from build123d import *

# Parameters (mm, degrees)
F0_R          = 8.875
F3_DEPTH      = 3
F3_DEPTH_BACK = 3
F4_SIZE       = 1
F5_R          = 0.5
F6_DEPTH      = 0.43


with BuildPart() as f2:
    # F0 (on Front) → F2 (revolve)
    with BuildSketch(Plane.XZ):
        with BuildLine():
            ThreePointArc((0, 10.375), (1.4661242569, 10.2708862647), (2.9028232275, 9.9606346339))
            ThreePointArc((2.9028232275, 9.9606346339), (9.4069705736, 10.9259285589), (15, 14.3833476682))
            Line((15, 14.3833476682), (3.7, 34.9606346339))
            Line((3.7, 34.9606346339), (0, 34.9606346339))
            Line((0, 34.9606346339), (0, 10.375))
        make_face()
    revolve(axis=Axis((0, 0, 0), (0, 0, 1)))

    # F0 (on Front) → F3 (join, two sides)
    with BuildSketch(Plane.XZ) as f3_sk:
        with BuildLine():
            ThreePointArc((0, 10.375), (-7.3362328548, -7.3362328548), (10.375, 0))
            ThreePointArc((10.375, 0), (8.2993197307, 6.2259069225), (2.9028232275, 9.9606346339))
            Line((2.9028232275, 9.9606346339), (0, 9.9606346339))
            Line((0, 9.9606346339), (0, 10.375))
        make_face()
        Circle(F0_R, mode=Mode.SUBTRACT)
        with BuildLine():
            Line((0, 9.9606346339), (2.9028232275, 9.9606346339))
            ThreePointArc((2.9028232275, 9.9606346339), (1.4661242569, 10.2708862647), (0, 10.375))
            Line((0, 10.375), (0, 9.9606346339))
        make_face()
    extrude(amount=F3_DEPTH)
    extrude(f3_sk.sketch, amount=-F3_DEPTH_BACK)

    # F4
    f4_edges = [f2.edges().sort_by_distance(p)[0] for p in [
        (-8.875, -3, 0),
        (-8.875, 3, 0),
    ]]
    chamfer(f4_edges, length=F4_SIZE)

    # F5 (on face) → F6 (cut)
    with BuildSketch(Plane.XY.offset(34.9606346339)):
        with BuildLine():
            ThreePointArc((0.0041443855, 1.7524251654), (-0.4908303614, 1.5473999123), (-0.6958556145, 1.0524251654))
            Line((-0.6958556145, 1.0524251654), (-0.6958556145, -1.0399995122))
            ThreePointArc((-0.6958556145, -1.0399995122), (-0.4908303614, -1.534974259), (0.0041443855, -1.7399995122))
            ThreePointArc((0.0041443855, -1.7399995122), (0.4991191323, -1.534974259), (0.7041443855, -1.0399995122))
            Line((0.7041443855, -1.0399995122), (0.7041443855, 1.0524251654))
            ThreePointArc((0.7041443855, 1.0524251654), (0.4991191323, 1.5473999123), (0.0041443855, 1.7524251654))
        make_face()
        with Locations((0.0021327037, 0.0014704808)):
            Circle(F5_R, mode=Mode.SUBTRACT)
        with BuildLine():
            ThreePointArc((-2.2493049037, 1.7524251654), (-2.7442796505, 1.5473999123), (-2.9493049037, 1.0524251654))
            Line((-2.9493049037, 1.0524251654), (-2.9493049037, -1.0399995122))
            ThreePointArc((-2.9493049037, -1.0399995122), (-2.7442796505, -1.534974259), (-2.2493049037, -1.7399995122))
            ThreePointArc((-2.2493049037, -1.7399995122), (-1.7543301568, -1.534974259), (-1.5493049037, -1.0399995122))
            Line((-1.5493049037, -1.0399995122), (-1.5493049037, 1.0524251654))
            ThreePointArc((-1.5493049037, 1.0524251654), (-1.7543301568, 1.5473999123), (-2.2493049037, 1.7524251654))
        make_face()
        with BuildLine():
            ThreePointArc((2.2571443855, 1.7524251654), (1.7621696386, 1.5473999123), (1.5571443855, 1.0524251654))
            Line((1.5571443855, 1.0524251654), (1.5571443855, -1.0399995122))
            ThreePointArc((1.5571443855, -1.0399995122), (1.7621696386, -1.534974259), (2.2571443855, -1.7399995122))
            ThreePointArc((2.2571443855, -1.7399995122), (2.7521191323, -1.534974259), (2.9571443855, -1.0399995122))
            Line((2.9571443855, -1.0399995122), (2.9571443855, 1.0524251654))
            ThreePointArc((2.9571443855, 1.0524251654), (2.7521191323, 1.5473999123), (2.2571443855, 1.7524251654))
        make_face()
    extrude(amount=-F6_DEPTH, mode=Mode.SUBTRACT)


solid = f2.part
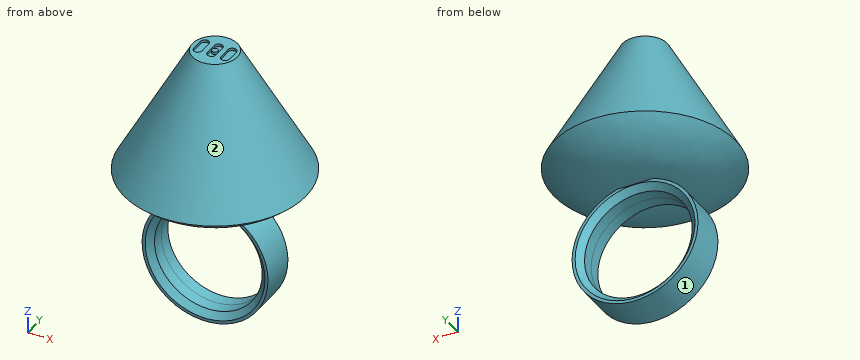
Could you check a few things on this model? Use its own coordinates, in mm. Face numbers are marked on the shaded views. Give positions to 0.01 mm unless a question says otherwise; leave off trailing zeros. Order: outer loops, then holes, each group sorted by start corner. A loop starts at its lowest first (then second) coordinate and runs counter-clockwise, first axis right, second up. Notation, with made-up numbers: (-28.75, 82) -> (19.25, 82) arc R13 cw to (19.25, 88) -> close; hole circle Ø5 at (45, -24). An arc over 180 degrees is marked (long way). Answer in a Markdown table with one row per item. Add a question column.
Item 1: Imagine slicing it at C-C (z = 27.5). List the corners of the cut face in (x, y) for me.
Item 2: Imagine slicing it at D-D (z = 15). List the corners of the cut face in (x, y) for me, and give its area (3 significant figures).
Item 3: Imagine slicing it at B-B (x = 5). Count the separate pieces of the cut face and the enclosed holes in it, and give its area (3 significant figures).
Item 4: I'm going to push flat-ended pins straight in: P1, Ø1, axis at x = -11.5, y = 7.5, coming from the -Z side; P2, Ø4, axis at y = 2, z = 20, coming from the +X side; P3, Ø5, axis at y = 7, z = 23, coming from the -X side. Where does each tip first touch, or does it pass through?
Item 5: Please list where these lines run through material, in increasing order: probe 1 along Z at (x, y) = (0, 0) (3 decimals); probe 2 along Z at (x, y) = (0, 1) (3 decimals); probe 3 along X at (y, z) = (-1, -5.5).
Item 6: We'd pull the mould along Z, two halves only. Please class the marked faces 1 and 2: pulls with the +Z half, pulls with the -Z half, needs draft (parallel to the pull), parting line crosses it, or undercut.
Item 7: Imagine slicing it at A-A (z = 0). List the corners of the cut face in (x, y) for me (3 decimals), and give its area (3 significant figures).
Result:
| question | item | result |
|---|---|---|
| 1 | outline | circle Ø15.59 at (0, 0) |
| 2 | outline | circle Ø29.32 at (0, 0) |
| 2 | area | 675 mm2 |
| 3 | separate pieces | 3 |
| 3 | enclosed holes | 0 |
| 3 | area | 416 mm2 |
| 4 | P1 | z = 12.93 |
| 4 | P2 | x = 12.89 |
| 4 | P3 | x = -9.95 |
| 5 | probe 1 | -10.375 to -8.875, 8.875 to 34.961 |
| 5 | probe 2 | -10.375 to -8.875, 8.875 to 34.531 |
| 5 | probe 3 | -8.8 to -6.97, 6.97 to 8.8 |
| 6 | face 1 | undercut |
| 6 | face 2 | pulls with the +Z half |
| 7 | outline | (-10.375, -3) -> (-9.875, -3) -> (-8.875, -2) -> (-8.875, 2) -> (-9.875, 3) -> (-10.375, 3) -> close; (8.875, -2) -> (9.875, -3) -> (10.375, -3) -> (10.375, 3) -> (9.875, 3) -> (8.875, 2) -> close |
| 7 | area | 16.0 mm2 |
